Part model, mm, in its own coordinate system. Give positions to 0.01 mm unless a question says otherwise; leave off trailing zeros. Order: outer loops, then holes, each group sorted by start corner. A loop starts at its lowest first (then second) coordinate and runs counter-clockwise, first axis right, second up. Notation, with made-up numbers: (46.5, 0.25) -> (72.5, 0.25) arc R16 ccw to (72.5, 6.25) -> close; hole circle Ø11 at (-35, 16). An arc over 180 degrees is marked (long way). Write item = value, one per line. Start each with the question number.
Item 1: Drill centre lines: line 1 along X through (y, z) = (1.1, 25.4); line 2 along X through (y, z) = (49, 25); line 3 along Z through (x, y) = (240, 21.5). Where is each one in solid material? Low to high.
Item 2: Band-saw the part on B-B on x = 62.5. Write the cut outline in (y, z).
Item 3: Band-saw the part on A-A on y = 26. Write the cut outline in (x, z).
```python
from build123d import *

# Parameters (mm, degrees)
BOSS_EXTRUDE1_DEPTH = 850.9
SKETCH2_R           = 4.7625
CUT_EXTRUDE1_DEPTH  = 850.9


with BuildPart() as part:
    # Sketch1 → Boss-Extrude1 (new body)
    with BuildSketch(Plane(origin=(0, 0, 0), x_dir=(0, 0, -1), z_dir=(1, 0, 0))):
        with BuildLine():
            Line((-6.35, 0), (-44.45, 0))
            ThreePointArc((-44.45, 0), (-48.940128061, 1.859871939), (-50.8, 6.35))
            Line((-50.8, 6.35), (-50.8, 44.45))
            ThreePointArc((-50.8, 44.45), (-48.940128061, 48.940128061), (-44.45, 50.8))
            Line((-44.45, 50.8), (-6.35, 50.8))
            ThreePointArc((-6.35, 50.8), (-1.859871939, 48.940128061), (0, 44.45))
            Line((0, 44.45), (0, 6.35))
            ThreePointArc((0, 6.35), (-1.859871939, 1.859871939), (-6.35, 0))
        make_face()
        with BuildLine():
            Line((-6.35, 4.699), (-44.45, 4.699))
            ThreePointArc((-44.45, 4.699), (-45.617433296, 5.182566704), (-46.101, 6.35))
            Line((-46.101, 6.35), (-46.101, 44.45))
            ThreePointArc((-46.101, 44.45), (-45.617433296, 45.617433296), (-44.45, 46.101))
            Line((-44.45, 46.101), (-6.35, 46.101))
            ThreePointArc((-6.35, 46.101), (-5.182566704, 45.617433296), (-4.699, 44.45))
            Line((-4.699, 44.45), (-4.699, 6.35))
            ThreePointArc((-4.699, 6.35), (-5.182566704, 5.182566704), (-6.35, 4.699))
        make_face(mode=Mode.SUBTRACT)
    extrude(amount=BOSS_EXTRUDE1_DEPTH)

    # Sketch2 → Cut-Extrude1 (cut)
    with BuildSketch(Plane(origin=(0, 50.8, 0), x_dir=(1, 0, 0), z_dir=(0, 1, 0))):
        with Locations(Location((38.1, -25.4, 0), (0, 0, 270))):
            Circle(SKETCH2_R)
        with Locations(Location((812.8, -25.4, 0), (0, 0, 270))):
            Circle(SKETCH2_R)
    extrude(amount=-CUT_EXTRUDE1_DEPTH, mode=Mode.SUBTRACT)


solid = part.part
```
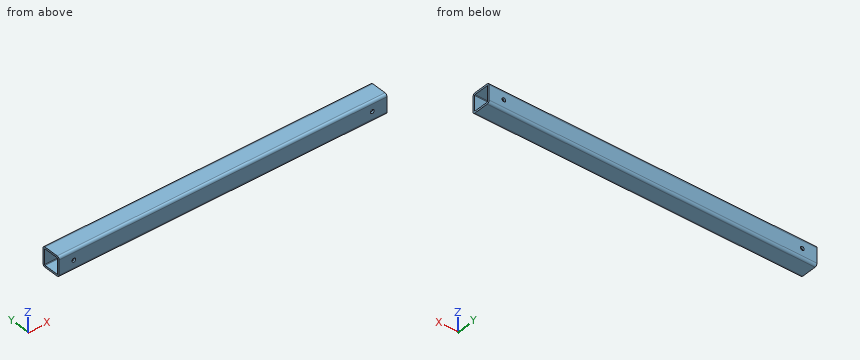
Values found:
q1.line_1 = 0 to 33.34, 42.86 to 808.04, 817.56 to 850.9
q1.line_2 = 0 to 33.35, 42.85 to 808.05, 817.55 to 850.9
q1.line_3 = 0 to 4.7, 46.1 to 50.8
q2.outline = (0, 6.35) arc R6.35 ccw to (6.35, 0) -> (44.45, 0) arc R6.35 ccw to (50.8, 6.35) -> (50.8, 44.45) arc R6.35 ccw to (44.45, 50.8) -> (6.35, 50.8) arc R6.35 ccw to (0, 44.45) -> close; hole (4.7, 6.35) arc R1.65 ccw to (6.35, 4.7) -> (44.45, 4.7) arc R1.65 ccw to (46.1, 6.35) -> (46.1, 44.45) arc R1.65 ccw to (44.45, 46.1) -> (6.35, 46.1) arc R1.65 ccw to (4.7, 44.45) -> close
q3.outline = (0, 0) -> (850.9, 0) -> (850.9, 4.7) -> (0, 4.7) -> close; (0, 46.1) -> (850.9, 46.1) -> (850.9, 50.8) -> (0, 50.8) -> close
